from build123d import *

# Parameters (mm, degrees)
SKETCH1_R           = 22.5
BOSS_EXTRUDE1_DEPTH = 150
CHAMFER1_SIZE       = 2
CUT_EXTRUDE6_DEPTH  = 90
CUT_EXTRUDE6_TAPER  = -0.57
CUT_EXTRUDE7_DEPTH  = 21


# Read off the part's stored shape, not the designer's step: Cut-Extrude6
with BuildPart() as part:
    # Sketch1 → Boss-Extrude1 (new body)
    with BuildSketch(Plane.XY):
        Circle(SKETCH1_R)
    extrude(amount=BOSS_EXTRUDE1_DEPTH)

    # Chamfer1
    chamfer1_edges = [part.edges().sort_by_distance(p)[0] for p in [
        (-22.5, 0, 150),
    ]]
    chamfer(chamfer1_edges, length=CHAMFER1_SIZE)

    # Cut-Extrude6 outline → Cut-Extrude6 (cut)
    with BuildSketch(Plane.XY.offset(60)):
        with BuildLine():
            ThreePointArc((6.104616555, 21.656030493), (5.946752148, 21.699911034), (5.788572381, 21.742640819))
            Line((5.788572381, 21.742640819), (-5.788572381, 21.742640819))
            ThreePointArc((-5.788572381, 21.742640819), (-5.946752148, 21.699911034), (-6.104616555, 21.656030493))
            Line((-6.104616555, 21.656030493), (-6.104616555, 20.645383445))
            Line((-6.104616555, 20.645383445), (6.104616555, 20.645383445))
            Line((6.104616555, 20.645383445), (6.104616555, 21.656030493))
        make_face()
    extrude(amount=CUT_EXTRUDE6_DEPTH, taper=CUT_EXTRUDE6_TAPER, mode=Mode.SUBTRACT)

    # Sketch6 → Cut-Extrude7 (cut)
    with BuildSketch(Plane(origin=(0, 21.240203456, 0.211312517), x_dir=(1, 0, 0), z_dir=(0, 0.9999505153082836, 0.009948212638374379))):
        Polygon((-6.98010259, -147.779884912), (6.98010259, -147.779884912), (6.104616555, -59.791646254), (-6.104616555, -59.781592122), align=None)
    extrude(amount=CUT_EXTRUDE7_DEPTH, mode=Mode.SUBTRACT)


solid = part.part
Check sheet for the modelled part. Datum: model origin and axes. Units: mm. Give positions to 0.01 mm unless a question says otherwise; leave off trailing zeros. Loops run counter-clockwise (first coordinate to the right, second up) from the corner with the lowest first, then second, coordinate; pieces in that order, holes last. Notation, with made-up numbers: M 32.5,84.5 L 85.5,84.5 A4 ccw 85.5,90.5 Z; hole C 75.5,79.25 d2. An arc over 180 degrees is marked long. Return JSON: item names as keys, results as strings. Group by question number.
1. Go/stop test with flat-tipped pins: pin 1 (8 mm diameter, centred on x = -12.5, z = 88.5, fed in from -Y); pin 2 (5 mm diameter, centred on y = 6.5, z = 52.5, fed in from -X); pin 3 (6 mm diameter, centred on x = -14, z = 25, fed in from +Y). Record where each tip stops, or that it passes through.
2. Cross-section at A-A on z = 20.5. Record the boundary of the cut face in (x, y), plus the area to 3 significant figures.
3. Thickness scan on L1, parallel to Y at x = 6.5, z = 135; L2, parallel to Y at x = -19, z = 103; L3, parallel to X at y = -3, z = 73. Record the ranges inside material, lowest first.
Return value:
{
 "1": {"pin 1": "y = -20.83", "pin 2": "x = -22.14", "pin 3": "y = 19.63"},
 "2": {"outline": "C 0,0 d45", "area": "1,590 mm^2"},
 "3": {"L1": "-21.54 to 19.9", "L2": "-12.05 to 12.05", "L3": "-22.3 to 22.3"}
}
